Source: CAD feature listing. Evaluate the final solid. Frame: model axes, mm. A direction names the side the tool comes from. Coordinates: 2 decimals unless noted, no trailing zeros. Order: outer loops, then holes, each group sorted by start corner. A loop starts at its lowest first (then second) coordinate and runs counter-clockwise, first axis right, second up.
Item 1: Ray query, line 1 (X direction, y = 27.5, z = 73); line 2 (Y direction, x = -10, z = 35); line 3 (Z direction, x = -23, y = -8). Return the intervals inside material, ascending.
Item 2: Section C-C on x = 21. Return the cut outline in (y, z).
Item 3: Mould query, pull axis X, two halves, no side actions, for faces 1 (the cylindrical face through (6.399, 24.451, 52.625)), 2 (the flat face through (17, 24, 87.884)), 3 (the flat face through (-27.709, 19, 34)). Classes: released by +X, released by -X, zero draft, split by the parting line, or undercut.
Item 4: Section D-D on z = 15. Return the cut outline in (x, y), then the cut area to 3 significant figures.
Item 5: Section A-A on z = 77. Return the cut outline in (x, y), then the cut area to 3 significant figures.
Item 6: Section B-B on y = 23.5. Return the cut outline in (x, z).
Item 7: Contact query for flat-ended pins moving along their axis: P1, Ø16, axis at x = 12, z = 46.5, coming from the -Y side; P2, Ø1.5, axis at x = -19, y = 3, coming from the +Z side; P3, Ø6.5, axis at x = 19, y = 23.5, coming from the -Z side. Output: stop coordinate, or through.
Item 8: Reachability of faces 4 (the flat face through (5, 17.895, 50)), 5 (the flat face through (9.944, 24, 74)), 6 (the flat face through (19, 24, 31.076)) from +Z, -Z, +X, -X, +Y, -Y: full face, straight path, thin tool, end or side. Return the list, or none.
from build123d import *

# Parameters (mm, degrees)
F1_DEPTH    = 25.4
F2_W        = 52.878184244
F2_H        = 12.9309091717
F3_DEPTH    = 87.884
F4_W        = 23.8667652011
F4_H        = 39.1564019587
F5_DEPTH    = 25.4
F6_T1_DEPTH = 12.9309091717
F8_DEPTH    = 12.954


# Not quite as in the source:
# - a fillet or chamfer that OpenCascade refuses, or shapes differently, is made with other operations: its cross-section is extruded or revolved along the edge and cut away or added


with BuildPart() as f1:
    # F0 (on Top) → F1 (new body)
    with BuildSketch(Plane.XY):
        with BuildLine():
            Line((25.1690931618, 17.8954545408), (-27.7090910822, 17.8954545408))
            Line((-27.7090910822, 17.8954545408), (-27.7090910822, -11.891817674))
            ThreePointArc((-27.7090910822, -11.891817674), (-1.2699989602, -23.9832848769), (25.1690931618, -11.891817674))
            Line((25.1690931618, -11.891817674), (25.1690931618, 17.8954545408))
        make_face()
    extrude(amount=F1_DEPTH)

    # F2 (on face) → F3 (join)
    with BuildSketch(Plane(origin=(0, 0, 0), x_dir=(1, 0, 0), z_dir=(0, 0, -1))):
        with Locations((-1.2699989602, -24.3609091267)):
            Rectangle(F2_W, F2_H)
    extrude(amount=-F3_DEPTH)

    # F4 (on face) → F5 (cut)
    with BuildSketch(Plane.XZ.offset(-17.8954545408)):
        with Locations((-1.9888961688, 68.3057990206)):
            Rectangle(F4_W, F4_H)
    extrude(amount=-F5_DEPTH, mode=Mode.SUBTRACT)

    # F6: fillet of radius 12.7 on 2 edges, made by hand

    # F6_s2 → F6_t1 (join)
    with BuildSketch(Plane.XZ.offset(-30.8263637125)):
        with BuildLine():
            ThreePointArc((-13.9222787693, 61.4275980413), (-10.2025348904, 52.4473419202), (-1.2222787693, 48.7275980413))
            Line((-1.2222787693, 48.7275980413), (-13.9222787693, 48.7275980413))
            Line((-13.9222787693, 48.7275980413), (-13.9222787693, 61.4275980413))
        make_face()
        with BuildLine():
            ThreePointArc((-2.7555135682, 48.7275980413), (6.2247425528, 52.4473419202), (9.9444864318, 61.4275980413))
            Line((9.9444864318, 61.4275980413), (9.9444864318, 48.7275980413))
            Line((9.9444864318, 48.7275980413), (-2.7555135682, 48.7275980413))
        make_face()
    extrude(amount=F6_T1_DEPTH)

    # F7 (on face) → F8 (cut)
    with BuildSketch(Plane.YZ.offset(25.1690931618)):
        Polygon((30.8263637125, 0), (30.8263637125, 31.0761313885), (17.8954545408, 31.0761313885), (17.8954545408, 25.4), (9.4672730193, 25.4), (9.4672730193, 0), align=None)
    extrude(amount=-F8_DEPTH, mode=Mode.SUBTRACT)


solid = f1.part
Answer list:
1. line 1: x = -27.71 to -13.92, 9.94 to 25.17
1. line 2: y = 17.9 to 30.83
1. line 3: z = 0 to 25.4
2. outline: (-15.97, 0) - (9.47, 0) - (9.47, 25.4) - (-15.97, 25.4) - close; (17.9, 31.08) - (30.83, 31.08) - (30.83, 87.88) - (17.9, 87.88) - close
3. face 1: undercut
3. face 2: zero draft
3. face 3: released by -X
4. outline: (-27.71, -11.89) arc R34.95 ccw to (25.17, -11.89) - (25.17, 9.47) - (12.22, 9.47) - (12.22, 30.83) - (-27.71, 30.83) - close
4. area: 2,430 mm2
5. outline: (-27.71, 17.9) - (-13.92, 17.9) - (-13.92, 30.83) - (-27.71, 30.83) - close; (9.94, 17.9) - (25.17, 17.9) - (25.17, 30.83) - (9.94, 30.83) - close
5. area: 375 mm2
6. outline: (-27.71, 0) - (12.22, 0) - (12.22, 31.08) - (25.17, 31.08) - (25.17, 87.88) - (9.94, 87.88) - (9.94, 61.43) arc R12.7 cw to (-1.99, 48.75) arc R12.7 cw to (-13.92, 61.43) - (-13.92, 87.88) - (-27.71, 87.88) - close
7. P1: stops at y = 17.9
7. P2: stops at z = 25.4
7. P3: stops at z = 31.08
8. face 4: +Z, +X, -X, -Y
8. face 5: +Z, +Y, -Y
8. face 6: -Z, +X, +Y, -Y
